Autodesk Inventor part; units mm, degrees
ref_plane "XZ Plane" through (0, 0, 0) normal (0, 1, 0) x (-1, 0, 0)
ref_plane "XY Plane" through (0, 0, 0) normal (0, 0, 1) x (1, 0, 0)
sketch "Sketch1" plane through (0, 0, 0) normal (0, 1, 0) x (-1, 0, 0)
  arc A0 (31.2876, -56.9744) -> (58.4216, -28.4941) centre (0, 0) ccw
  line L0 (0, -76.4247) -> (0, 75.7077)
  line L1 (75.2776, 0) -> (-75.7077, 0)
  line L2 (0, 0) -> (78.1118, -78.1118)
  line L3 (0, 0) -> (84.1598, -41.0475)
  line L4 (0, 0) -> (41.0475, -84.1598)
  circle A1 centre (38.0152, -38.0152) radius 2
  arc A2 (40.7893, -32.7712) -> (32.7712, -40.7893) centre (38.0152, -38.0152) ccw
  line L5 (27.1472, -55.66) -> (27.0904, -55.5436)
  arc A3 (27.1472, -55.66) -> (31.2876, -56.9744) centre (29.8436, -54.3448) ccw
  arc A4 (28.4686, -51.5336) -> (27.0904, -55.5436) centre (29.7868, -54.2284) ccw
  arc A5 (28.4686, -51.5336) -> (29.2312, -51.1337) centre (-5.4867, 14.1516) ccw
  line L6 (32.7449, -40.7314) -> (32.4923, -40.1813)
  arc A6 (29.2312, -51.1337) -> (32.7449, -40.7314) centre (25.475, -44.0703) ccw
  line L7 (55.66, -27.1472) -> (55.5436, -27.0904)
  arc A7 (56.9744, -31.2876) -> (55.66, -27.1472) centre (54.3448, -29.8436) ccw
  arc A8 (55.5436, -27.0904) -> (51.5336, -28.4686) centre (54.2284, -29.7868) ccw
  arc A9 (51.1337, -29.2312) -> (51.5336, -28.4686) centre (-14.1516, 5.4867) ccw
  arc A10 (40.7314, -32.7449) -> (51.1337, -29.2312) centre (44.0703, -25.475) ccw
  point P0 (28.4941, -58.4216)
  point P1 (25.6079, -52.5039)
  point P2 (35.7325, -47.2364)
  point P3 (55.5436, -27.0904)
  dimension "d0" = 65
  dimension "d1" = 45
  dimension "d2" = 26
  dimension "d3" = 4
  dimension "d4" = 3
  dimension "d6" = 8
extrude "Extrusion1" add sketch "Sketch1" along normal blind 30 contours A0 L2 A1 A2 A10 A9 A8 L3 A7 | A0 A3 L4 A4 A5 A6 L6 A2 L2 A1
ref_plane "Work Plane1" through (0, 0, 0) normal (0.7071, 0, -0.7071) x (0, 1, 0)
properties part number "Foam Attachment"
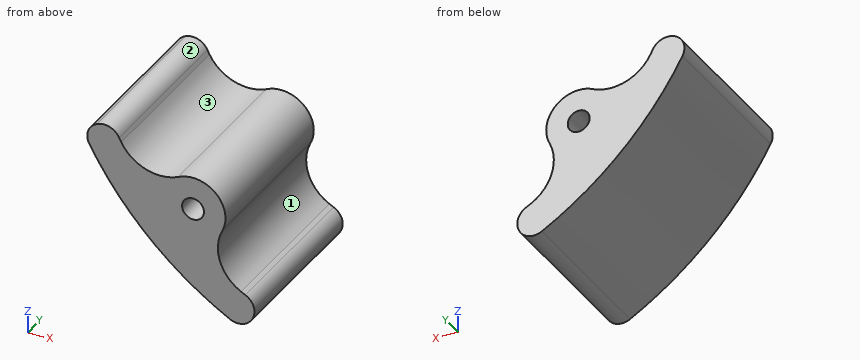
Work out the finished part from the listing and answer in its coordinate system (mm). Face numbers are marked on the shaded views. Coordinates: 2 decimals unless noted, no trailing zeros. Loops run counter-clockwise (first coordinate to the right, second up) from the corner with the lowest first, then second, coordinate; pieces in that order, holes last.
1) For a pull along X with two mould halves and no side action, classify the marked faces 1, 2 and 3 as +X half, -X half, draft (parallel to the pull), parting line (faces both ways), or undercut.
Results:
face 1: +X half
face 2: parting line
face 3: undercut
2) Section D-D (x = -35) is taken. Give the vertices of the cut face in (y, z), plus the area to 3 significant figures.
Results:
outline: (0, -54.77) - (30, -54.77) - (30, -32.91) - (0, -32.91) - close
area: 656 mm2
3) Consider probe 1 along Z at (x, y) = (-38.5, 4.25); probe 2 along Z at (x, y) = (-39, 3); probe 3 along X at (y, z) = (21, -46). Determine where each line is inside the solid, lowest interval first.
Results:
probe 1: z = -52.37 to -39.96, -36.07 to -32.1
probe 2: z = -52 to -39.76, -36.27 to -32.16
probe 3: x = -45.92 to -33.24
4) Section C-C (z = -54) is taken. Give the vertices of the cut face in (x, y), plus the area to 3 significant figures.
Results:
outline: (-36.18, 0) - (-26.8, 0) - (-26.8, 30) - (-36.18, 30) - close
area: 282 mm2
5) Flat-ended cylindrical pins translate along their axes: pin 1 (4 mm diameter, centred on x = -35, z = -54, fed in from -Y); pin 2 (10 mm diameter, centred on x = -36, y = 15.5, fed in from -Z); pin 3 (3 mm diameter, centred on y = 25.5, z = -45.5, fed in from -X); pin 4 (2 mm diameter, centred on x = -32, y = 12, fed in from +Z). Find the tip coordinate at first contact, or state that the pin passes through.
Results:
pin 1: stops at y = 0
pin 2: stops at z = -57.11
pin 3: stops at x = -47.84
pin 4: stops at z = -34.85
6) Section A-A (x = -39.5) is taken. Give the vertices of the cut face in (y, z).
Results:
outline: (0, -51.62) - (30, -51.62) - (30, -39.36) - (0, -39.36) - close; (0, -36.68) - (30, -36.68) - (30, -32.27) - (0, -32.27) - close
7) Section B-B (y = 10.25) is taken. Give the vertices of the cut face in (x, z).
Results:
outline: (-56.97, -31.29) arc R65 ccw to (-31.29, -56.97) arc R3 ccw to (-27.15, -55.66) - (-27.09, -55.54) arc R3 ccw to (-28.47, -51.53) arc R72.97 cw to (-29.23, -51.13) arc R8 cw to (-32.74, -40.73) - (-32.49, -40.18) arc R5.93 ccw to (-40.79, -32.77) arc R8 cw to (-51.13, -29.23) arc R74.94 cw to (-51.53, -28.47) arc R3 ccw to (-55.54, -27.09) - (-55.66, -27.15) arc R3 ccw to start; hole circle Ø4 at (-38.02, -38.02)
